Autodesk Inventor part; units mm, degrees
ref_plane "YZ Plane" through (0, 0, 0) normal (1, 0, 0) x (0, 1, 0)
ref_plane "XZ Plane" through (0, 0, 0) normal (0, 1, 0) x (-1, 0, 0)
ref_plane "XY Plane" through (0, 0, 0) normal (0, 0, 1) x (1, 0, 0)
sketch "Sketch1" plane through (0, 0, 0) normal (1, 0, 0) x (0, 1, 0)
  line L0 (52.3875, 0) -> (52.3875, 2)
  line L1 (52.3875, 0) -> (52.3875, -2)
  arc A0 (52.3875, 2) -> (50.9047, 4.0295) centre (50.2572, 2) ccw
  arc A1 (51.1141, -2.9824) -> (52.3875, -2) centre (51.3718, -2) ccw
  line L2 (50.9047, 4.0295) -> (25.8188, 7.012) construction
  line L3 (25.8188, 7.012) -> (16.2938, 5.4245) construction
  line L4 (16.2938, 5.4245) -> (-0.0182, 1.08) construction
  spline S0 degree 3 poles (50.9047, 4.0295) (25.8188, 7.012) (16.2938, 5.4245) (-0.0182, 1.08) knots 1 1 1 1 2 2 2 2
  line L5 (0, 0) -> (52.3875, 0)
  line L6 (51.1141, -2.9824) -> (25.8188, -7.012) construction
  line L7 (25.8188, -7.012) -> (16.2938, -5.4245) construction
  line L8 (16.2938, -5.4245) -> (-0.0182, -1.08) construction
  spline S1 degree 3 poles (51.1141, -2.9824) (25.8188, -7.012) (16.2938, -5.4245) (-0.0182, -1.08) knots 1 1 1 1 2 2 2 2
  line L9 (-0.0182, -1.08) -> (-0.0182, 1.08)
  dimension "d0" = 2
  dimension "d1" = 2
revolve "Revolution1" add sketch "Sketch1" angle 360 about axis through (0, -0.0182, -1.08) along (0, 0, 1)
sketch "Sketch2" plane through (0, 0, 0) normal (0, 0, 1) x (1, 0, 0)
  circle A0 centre (0, 0) radius 6.35
extrude "Extrusion1" cut sketch "Sketch2" along normal mid plane 105.25
sketch "Sketch3" plane through (0, 0, 0) normal (0, 0, 1) x (1, 0, 0)
  line L0 (0, 0) -> (-14.2875, -39.6875)
  arc A0 (-14.2875, -39.6875) -> (12.7, -39.6875) centre (-0.7937, -2.2049) ccw
  line L1 (12.7, -39.6875) -> (0, 0)
  line L2 (0, 0) -> (-6.2667, -17.4074)
  line L3 (5.588, -17.4625) -> (0, 0)
  arc A1 (5.588, -17.4625) -> (-6.2667, -17.4074) centre (-0.3491, -19.5378) ccw
  line L4 (39.6875, 12.7) -> (0, 0)
  arc A2 (39.6875, -14.2875) -> (39.6875, 12.7) centre (2.2049, -0.7937) ccw
  line L5 (0, 0) -> (39.6875, -14.2875)
  arc A3 (17.4625, 5.588) -> (17.4074, -6.2667) centre (19.5378, -0.3491) ccw
  line L6 (-12.7, 39.6875) -> (0, 0)
  arc A4 (14.2875, 39.6875) -> (-12.7, 39.6875) centre (0.7937, 2.2049) ccw
  line L7 (0, 0) -> (14.2875, 39.6875)
  arc A5 (-5.588, 17.4625) -> (6.2667, 17.4074) centre (0.3491, 19.5378) ccw
  line L8 (-39.6875, -12.7) -> (0, 0)
  arc A6 (-39.6875, 14.2875) -> (-39.6875, -12.7) centre (-2.2049, 0.7938) ccw
  line L9 (0, 0) -> (-39.6875, 14.2875)
  arc A7 (-17.4625, -5.588) -> (-17.4074, 6.2667) centre (-19.5378, 0.3491) ccw
  dimension "d13" = 360
extrude "Extrusion3" cut sketch "Sketch3" along normal mid plane 105.25 contours A1 L1 A0 L0 | L4 A2 L5 A3 | L6 A4 L7 A5 | L8 A6 L9 A7
properties part number "Anti tip wheels"
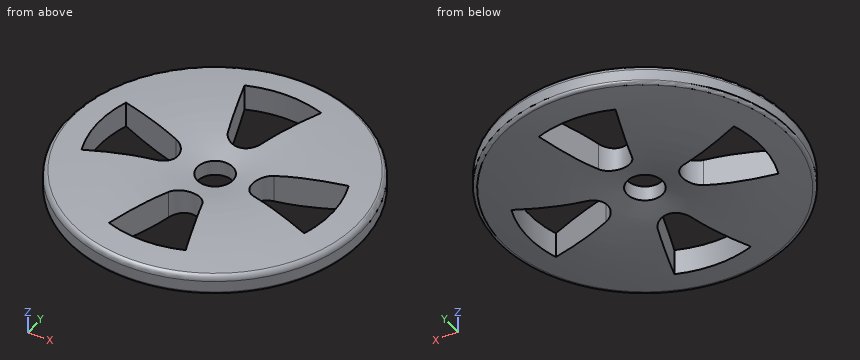
Verification items for the finished model (mm, model axes). Round coordinates to 2 decimals unless told otherwise and drop trailing zeros. Write each loop counter-clockwise with the first axis right and the second up, starting at its lowest first coordinate (ties: lowest second). Pieces come first, ordered by that corner, then holes.
(1) Material ranges on line 1 (X direction, y = 0, z = -0.95); line 2 (Y direction, x = 0, z = 1.35); line 3 (X direction, y = -4.5, z = 2.25), recorded low to high.
Returned:
line 1: x = -52.41 to -42.03, -13.26 to -6.35, 6.35 to 13.26, 42.03 to 52.41
line 2: y = -52.42 to -42.03, -13.26 to -6.35, 6.35 to 13.26, 42.03 to 52.39
line 3: x = -52.2 to -41.69, -15.53 to -4.48, 4.48 to 14.81, 41.87 to 52.2
(2) Depth check by flat-ended pin: pin 1 Ø20.5 at (x, y) = (0, 0) entering from -Z; pin 2 Ø4 at (x, z) = (-38.5, -1.5) entering from -Y; pin 3 Ø5 at (x, z) = (27.5, -1.5) entering from +Y. Enter the tip coordinate at first touch or a pass-through.
Returned:
pin 1: stops at z = -3.57
pin 2: stops at y = -37.62
pin 3: stops at y = 46.04
(3) Section check A-A (z = 0.5). Enter the section's corners in (x, y).
Returned:
outline: circle Ø104.81 at (0, -0.02); hole (-39.69, -12.7) - (-17.46, -5.59) arc R6.29 ccw to (-17.41, 6.27) - (-39.69, 14.29) arc R39.84 ccw to start; hole (-14.29, -39.69) arc R39.84 ccw to (12.7, -39.69) - (5.59, -17.46) arc R6.29 ccw to (-6.27, -17.41) - close; hole (-12.7, 39.69) - (-5.59, 17.46) arc R6.29 ccw to (6.27, 17.41) - (14.29, 39.69) arc R39.84 ccw to start; hole circle Ø12.7 at (0, 0); hole (17.41, -6.27) - (39.69, -14.29) arc R39.84 ccw to (39.69, 12.7) - (17.46, 5.59) arc R6.29 ccw to start
(4) Section check B-B (x = 0). Give the number of separate pieces and of enclosed holes in the cut face, plus the area to 3 significant figures.
Returned:
separate pieces: 4
enclosed holes: 0
area: 260 mm2
